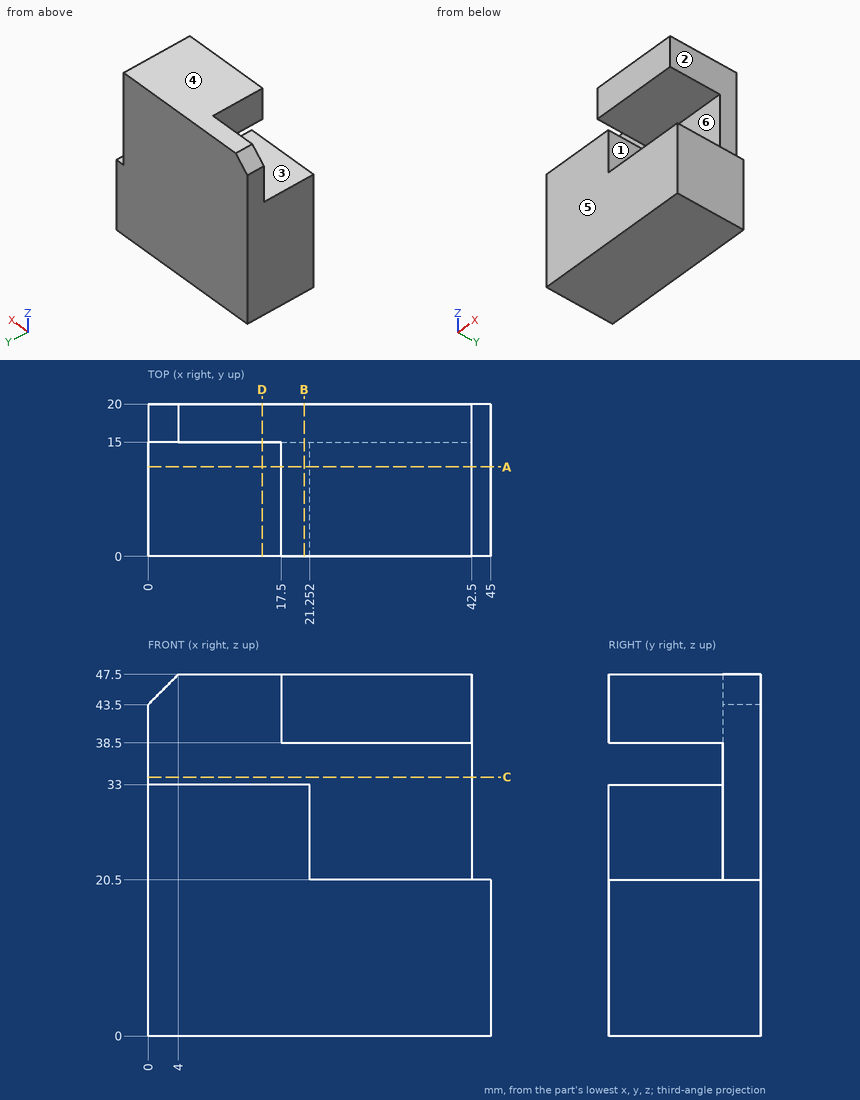
Verification items for this drawing (mm, ordinates from the low corner). A direction names the side the tool comes from. Coordinates: 2 decimals unless noted, no trailing zeros. Order: outer loops, then holes, each group sorted by start corner. A loop starts at its lowest first (then second) coordinate and runs counter-clockwise, first axis right, second up. Notation, with made-up numbers: (18, 81) - (39, 81) arc R21 ccw to (39, 95) - close; hole circle Ø2 at (4.25, 39.25). An arc over 180 degrees is marked (long way). Answer in a Markdown table with one row per item. Add a question column.
1. Section check A-A (y = 11.75). Enter the section's corners in (x, z), plus the area to 3 significant figures.
2. Section check B-B (x = 20.5). Enter the section's corners in (y, z).
3. Draft check along Z on the marked faces 4, 5 and 6. Enter one of: +Z half, -Z half, draft (parallel to the pull), parting line (faces both ways), or undercut.
4. Gauge pin test, flat ends, axial feed: pin 1 Ø8 at (x, z) = (30.5, 32) entering from -Y; pin 2 Ø10 at (y, z) = (11, 29) entering from +X; pin 3 Ø4.5 at (y, z) = (7, 43) entering from -X. Record the tip position at first contact, or that the pin passes through.
5. Access from +Z, -Z, +X, -X, +Y, -Y to the whole of each face (thin tool, end or side, straight path). Record for the marked faces 1, 2 and 3.
6. Section check C-C (z = 34). Enter the section's corners in (x, y).
7. Material ranges on L1, parallel to Z at x = 24, y = 14; L2, parallel to X at y = 2.5, z = 44; L3, parallel to Z at x = 20, y = 5.75, recorded low to high. Write a range as [from, to].
8. Section check D-D (x = 15). Enter the section's corners in (y, z).
Data:
| question | item | result |
|---|---|---|
| 1 | outline | (0, 0) - (45, 0) - (45, 20.5) - (21.25, 20.5) - (21.25, 33) - (0, 33) - close; (17.5, 38.5) - (42.5, 38.5) - (42.5, 47.5) - (17.5, 47.5) - close |
| 1 | area | 1,410 mm² |
| 2 | outline | (0, 0) - (20, 0) - (20, 47.5) - (0, 47.5) - (0, 38.5) - (15, 38.5) - (15, 33) - (0, 33) - close |
| 3 | face 4 | +Z half |
| 3 | face 5 | draft |
| 3 | face 6 | undercut |
| 4 | pin 1 | stops at y = 15 |
| 4 | pin 2 | stops at x = 42.5 |
| 4 | pin 3 | stops at x = 17.5 |
| 5 | face 1 | +X, -Y |
| 5 | face 2 | +Z, +X, +Y, -Y |
| 5 | face 3 | +X, -X, -Y |
| 6 | outline | (0, 15) - (42.5, 15) - (42.5, 20) - (0, 20) - close |
| 7 | L1 | z = [0, 20.5], [38.5, 47.5] |
| 7 | L2 | x = [17.5, 42.5] |
| 7 | L3 | z = [0, 33], [38.5, 47.5] |
| 8 | outline | (0, 0) - (20, 0) - (20, 47.5) - (15, 47.5) - (15, 33) - (0, 33) - close |
